The model under review builds one solid part; all positions refer to its coordinate system, in mm. Round coordinates to 2 decimals unless told otherwise and drop trailing zeros. Order: outer loops, then holes, each group sorted by start corner. A loop starts at its lowest first (then second) coordinate and runs counter-clockwise, first axis right, second up. Notation, with made-up numbers: (-5, 41.25) - (3, 41.25) arc R21 ccw to (3, 76.25) - close; hole circle Ø10 at (-6.75, 27). An arc over 180 degrees is marked (long way). One line per question, with ' | ' between items. Start each with the question number.
Item 1: Add section A-A on x = 6.5. State the section outline as (y, z) points.
Item 2: Add section B-B on z = 13.5. State the section outline as (x, y) points, and give its area (3 significant figures).
Item 3: Add section C-C on y = -5. State the section outline as (x, z) points.
Item 4: Draft analysis for pull direction X (two halves, no side actions). For faces 1 (the face through (6, -6, -18.04)), 2 (the face through (31.845, -6, 7)), 3 (the face through (4.974, -6.261, 20.483)), state which applies: +X half, -X half, draft (parallel to the pull), parting line (faces both ways), or undercut.
Item 5: For L1, parallel to Z at x = 6.5, y = -1.5; L2, parallel to Z at x = 1, y = -6.5; L3, parallel to X at y = -4, z = 2, list the stretches that pass through material, from the lowest coordinate up. Write a range as [from, to].
from build123d import *

# Parameters (mm, degrees)
F0_W     = 50.8
F0_H     = 50.8
F0_R     = 11.298879
F1_DEPTH = 12.7
F2_DEPTH = 12.7


with BuildPart() as f1:
    # F0 (on Front) → F1 (new body)
    with BuildSketch(Plane.XZ):
        with Locations((6.445251, 7.359565)):
            Rectangle(F0_W, F0_H)
        with Locations((6.445251, 9.280269)):
            Circle(F0_R, mode=Mode.SUBTRACT)
    extrude(amount=F1_DEPTH)

    # F0 (on Front) → F2 (join)
    with BuildSketch(Plane.XZ):
        with Locations((6.445251, 7.359565)):
            Rectangle(F0_W, F0_H)
        with Locations((6.445251, 9.280269)):
            Circle(F0_R, mode=Mode.SUBTRACT)
    extrude(amount=F2_DEPTH)


solid = f1.part
Determined:
1) outline: (-12.7, -18.04) - (0, -18.04) - (0, -2.02) - (-12.7, -2.02) - close; (-12.7, 20.58) - (0, 20.58) - (0, 32.76) - (-12.7, 32.76) - close
2) outline: (-18.95, -12.7) - (-4.04, -12.7) - (-4.04, 0) - (-18.95, 0) - close; (16.93, -12.7) - (31.85, -12.7) - (31.85, 0) - (16.93, 0) - close | area: 379 mm2
3) outline: (-18.95, -18.04) - (31.85, -18.04) - (31.85, 32.76) - (-18.95, 32.76) - close; hole circle Ø22.6 at (6.45, 9.28)
4) face 1: draft | face 2: +X half | face 3: undercut
5) L1: [-18.04, -2.02], [20.58, 32.76] | L2: [-18.04, -0.62], [19.18, 32.76] | L3: [-18.95, -2.2], [15.09, 31.85]
